from build123d import *

# Parameters (mm, degrees)
F0_W     = 152.4
F0_H     = 57.531
F1_DEPTH = 6.35
F2_W     = 101.6
F2_H     = 57.531
F3_DEPTH = 101.6
F4_F1_R  = 6.35
F4_F2_R  = 6.3499


# Not quite as in the source:
# - a fillet or chamfer is up to 0.001 mm smaller than in the source, because OpenCascade refuses the exact size


with BuildPart() as f1:
    # F0 (on Front) → F1 (new body)
    with BuildSketch(Plane.XZ):
        Rectangle(F0_W, F0_H)
    extrude(amount=F1_DEPTH)

    # F2 (on face) → F3 (join)
    with BuildSketch(Plane.XZ.offset(6.35)):
        Rectangle(F2_W, F2_H)
    extrude(amount=F3_DEPTH)

    # F4: fillet of radius 6.35 on 11 edges, made by hand

    # F4_f1
    f4_f1_edges = [f1.edges().sort_by_distance(p)[0] for p in [
        (50.8, -6.35, 0),
        (-50.8, -6.35, 0),
    ]]
    fillet(f4_f1_edges, radius=F4_F1_R)

    # F4_f2 (radius 6.35 in the source; OpenCascade refuses exactly that, so slightly less here)
    f4_f2_edges = [f1.edges().sort_by_distance(p)[0] for p in [
        (-76.2, -3.175, -28.7655),
        (-50.8, -60.325, -28.7655),
        (-50.8, -60.325, 28.7655),
        (50.8, -60.325, -28.7655),
        (50.8, -60.325, 28.7655),
        (-50.8, -107.95, 0),
        (-76.2, -3.175, 28.7655),
        (76.2, -3.175, 28.7655),
        (76.2, -3.175, -28.7655),
        (52.6598719395, -8.2098719395, 28.7655),
        (52.6598719395, -8.2098719395, -28.7655),
        (-52.6598719395, -8.2098719395, 28.7655),
        (-52.6598719395, -8.2098719395, -28.7655),
    ]]
    fillet(f4_f2_edges, radius=F4_F2_R)


solid = f1.part
CAD build for the part. Positions are in the model's coordinates, mm. A direction names the side the tool comes from. Round coordinates to 2 decimals unless told otherwise and drop trailing zeros. Loops run counter-clockwise (first coordinate to the right, second up) from the corner with the lowest first, then second, coordinate; pieces in that order, holes last.
(1) Cut at B-B (z = -5). Give the cut face in (x, y), plus the area to 3 significant figures.
(2) Which spindle directions (+Z, -Z, +X, -X, +Y, -Y) get a long thin tool onto all of the face, cutting with end or side? Do faces 1 (the flat face through (-50.8, -57, 0)), 2 (the cylindrical face through (-66.542, -4.441, -26.955)), 3 (the cylindrical face through (-66.542, -4.539, 26.856)). Say none if no direction does.
(3) Wall check: line 1 along X through (y, z) = (-67.5, -17); line 2 along Y through (x, z) = (-66, 13); line 3 along X through (y, z) = (-70, 26). Give the ranges that are in metal, low to high.
(4) Drop flat-ended pins along their axis: pin 1 (8 mm diameter, centred on y = -73.5, z = -15, fed in from +X); pin 2 (2 mm diameter, centred on x = 55.5, z = -13.5, fed in from +Y); pin 3 (5.5 mm diameter, centred on x = -70, z = 9, fed in from -Y); pin 4 (2 mm diameter, centred on y = -97, z = -21, fed in from -X). Give the stop position or say it passes through.
(5) Cut at A-A (y = -67). Give the cut face in (x, z), plus the area to 3 significant figures.
Findings below:
1. outline: (-76.2, -6.35) - (-57.15, -6.35) arc R6.35 cw to (-50.8, -12.7) - (-50.8, -101.6) arc R6.35 ccw to (-44.45, -107.95) - (50.8, -107.95) - (50.8, -12.7) arc R6.35 cw to (57.15, -6.35) - (76.2, -6.35) - (76.2, 0) - (-76.2, 0) - close
1. area: 11,300 mm2
2. face 1: +Z, -Z, -X, -Y
2. face 2: -Z, -X, -Y
2. face 3: +Z, -X, -Y
3. line 1: x = -50.8 to 50.8
3. line 2: y = -6.35 to 0
3. line 3: x = -49.69 to 49.69
4. pin 1: stops at x = 50.8
4. pin 2: stops at y = 0
4. pin 3: stops at y = -6.35
4. pin 4: stops at x = -50.8
5. outline: (-50.8, -22.42) arc R6.35 ccw to (-44.45, -28.77) - (44.45, -28.77) arc R6.35 ccw to (50.8, -22.42) - (50.8, 22.42) arc R6.35 ccw to (44.45, 28.77) - (-44.45, 28.77) arc R6.35 ccw to (-50.8, 22.42) - close
5. area: 5,810 mm2
